Geometry check sheet. Reference: the model listing, model coordinates, mm. A direction names the side the tool comes from. Coordinates: 2 decimals unless noted, no trailing zeros. Write each loop counter-clockwise with the first axis right and the second up, starting at its lowest first coordinate (ties: lowest second). Pieces come first, ordered by that corner, then holes. Notation, with made-up numbers: (-1, -24) -> (14, -24) arc R36 cw to (14, 14) -> close; hole circle Ø2 at (-14.75, 61). An arc over 180 degrees is marked (long way). Use a Markdown table: item, result.
```python
from build123d import *

# Parameters (mm, degrees)
SKETCH_1_R              = 40
SKETCH_1_R_2            = 13.5
EXTRUDE_1_DEPTH         = 2
HOLE_WIZARD_M4_1_D      = 4.5
HOLE_WIZARD_5_4_5_4_1_D = 5.4
SKETCH_8_R              = 29.5
SKETCH_8_R_2            = 21.5
EXTRUDE_2_DEPTH         = 29
CUT_EXTRUDE_START       = -9
SKETCH_10_R             = 29.5
SKETCH_10_R_2           = 27.5
CUT_EXTRUDE_2_DEPTH     = 9
HOLE_WIZARD_M3_1_D      = 2.5
HOLE_WIZARD_M3_1_DEPTH  = 8.5
HOLE_WIZARD_M3_1_TIP    = 0.751075774


with BuildPart() as part:
    # 草图1 → 凸台-拉伸1 (new body)
    with BuildSketch(Plane.XY):
        Circle(SKETCH_1_R)
        Circle(SKETCH_1_R_2, mode=Mode.SUBTRACT)
    extrude(amount=EXTRUDE_1_DEPTH)

    # M4 间隙孔1 (through all)
    with Locations(Plane(origin=(-17.5, 0, 2), x_dir=(1, 0, 0), z_dir=(0, 0, 1))):
        with Locations((0, 0), (17.5, 17.5), (35, 0), (17.5, -17.5)):
            Hole(HOLE_WIZARD_M4_1_D / 2)

    # Ø5.4 (5.4) 直径孔1 (through all)
    with Locations(Plane(origin=(0, 0, 0), x_dir=(-1, 0, 0), z_dir=(0, 0, -1))):
        with Locations((-30.310889132, 17.5), (0, 35), (30.310889132, 17.5), (30.310889132, -17.5), (0, -35), (-30.310889132, -17.5)):
            Hole(HOLE_WIZARD_5_4_5_4_1_D / 2)

    # 草图8 → 凸台-拉伸2 (add)
    with BuildSketch(Plane(origin=(0, 0, 0), x_dir=(-1, 0, 0), z_dir=(0, 0, -1))):
        with Locations(Location((0, 0, 0), (0, 0, 180))):
            Circle(SKETCH_8_R)
        with Locations(Location((0, 0, 0), (0, 0, 180))):
            Circle(SKETCH_8_R_2, mode=Mode.SUBTRACT)
    extrude(amount=EXTRUDE_2_DEPTH)

    # 草图10 → 切除-拉伸2 (cut)
    with BuildSketch(Plane(origin=(0, 0, -29), x_dir=(-1, 0, 0), z_dir=(0, 0, -1)).offset(CUT_EXTRUDE_START)):
        with Locations(Location((0, 0, 0), (0, 0, 180))):
            Circle(SKETCH_10_R)
        Circle(SKETCH_10_R_2, mode=Mode.SUBTRACT)
    extrude(amount=CUT_EXTRUDE_2_DEPTH, mode=Mode.SUBTRACT)

    # M3 螺纹孔1
    with Locations(Plane(origin=(25, 0, -29), x_dir=(-1, 0, 0), z_dir=(0, 0, -1))):
        with Locations((0, 0), (25, 25), (50, 0), (25, -25)):
            Hole(HOLE_WIZARD_M3_1_D / 2, depth=HOLE_WIZARD_M3_1_DEPTH)
            with Locations((0, 0, -(HOLE_WIZARD_M3_1_DEPTH + HOLE_WIZARD_M3_1_TIP / 2))):  # 118° drill point
                Cone(0, HOLE_WIZARD_M3_1_D / 2, HOLE_WIZARD_M3_1_TIP, mode=Mode.SUBTRACT)


solid = part.part
```
Item 1: Depth check by flat-ended pin: P1, Ø5, axis at y = -21.5, z = -21, coming from the -X side; P2, Ø6, axis at x = 17.5, y = 0, coming from the -Z side; P3, Ø1.5, axis at y = -15, z = -10.5, coming from the -X side. Enter the tip coordinate at first touch or a pass-through.
Answer block:
| item | result |
|---|---|
| P1 | stops at x = -22.39 |
| P2 | stops at z = 0 |
| P3 | stops at x = -25.83 |
Item 2: Section check B-B on y = 34. Record the boundary of the cut face in (x, z).
Answer block:
| item | result |
|---|---|
| outline | (-21.07, 0) -> (-2.51, 0) -> (-2.51, 2) -> (-21.07, 2) -> close; (2.51, 0) -> (21.07, 0) -> (21.07, 2) -> (2.51, 2) -> close |
Item 3: Tool access check on faces 1 (the cylindrical face through (-23.845, -0.479, -24.69)), 2 (the flat face through (14.13, -16.42, -29)). Record the directions out of +Z, -Z, +X, -X, +Y, -Y that give a thin tool (end or side, any length) a straight path to the whole face; none if there is none.
Answer block:
| item | result |
|---|---|
| face 1 | -Z |
| face 2 | -Z, +X, -X, +Y, -Y |
Item 4: Thickness scan on L1, parallel to Y at x = 0, z = -26.5; L2, parallel to Y at x = 9.5, z = -13; L3, parallel to Y at x = 2, z = -21. Record the ranges inside material, lowest first. Write a range as [from, to].
Answer block:
| item | result |
|---|---|
| L1 | y = [-27.5, -26.25], [-23.75, -21.5], [21.5, 23.75], [26.25, 27.5] |
| L2 | y = [-27.93, -19.29], [19.29, 27.93] |
| L3 | y = [-27.43, -21.41], [21.41, 27.43] |
Item 5: Mould release check, pull along Y, two halves, no side actions. Record for faces 3 (the cylindrical face through (-28.9, -15.2, 1)), 4 (the flat face through (17, -8, 2)), 5 (the cylindrical face through (28.14, -8.86, -9.86)), 6 (the cylindrical face through (-2.93, -13.18, 0.99)): +Y half, -Y half, draft (parallel to the pull), parting line (faces both ways), or undercut.
Answer block:
| item | result |
|---|---|
| face 3 | undercut |
| face 4 | draft |
| face 5 | parting line |
| face 6 | undercut |
Item 6: Section check C-C on z = -11. Record the boundary of the cut face in (x, y), then the cut area to 3 significant figures.
Answer block:
| item | result |
|---|---|
| outline | circle Ø59 at (0, 0); hole circle Ø43 at (0, 0) |
| area | 1,280 mm^2 |
Item 7: Section check D-D on y = -17.5. Record the boundary of the cut face in (x, z), then the cut area to 3 significant figures.
Answer block:
| item | result |
|---|---|
| outline | (-35.97, 0) -> (-33.01, 0) -> (-33.01, 2) -> (-35.97, 2) -> close; (-27.61, 0) -> (-23.75, 0) -> (-23.75, -20) -> (-21.21, -20) -> (-21.21, -29) -> (-12.49, -29) -> (-12.49, 0) -> (-2.25, 0) -> (-2.25, 2) -> (-27.61, 2) -> close; (2.25, 0) -> (12.49, 0) -> (12.49, -29) -> (21.21, -29) -> (21.21, -20) -> (23.75, -20) -> (23.75, 0) -> (27.61, 0) -> (27.61, 2) -> (2.25, 2) -> close; (33.01, 0) -> (35.97, 0) -> (35.97, 2) -> (33.01, 2) -> close |
| area | 721 mm^2 |
Item 8: Section check A-A on x = -17.5. Record the boundary of the cut face in (y, z), then the cut area to 3 significant figures.
Answer block:
| item | result |
|---|---|
| outline | (-35.97, 0) -> (-23.75, 0) -> (-23.75, -20) -> (-21.21, -20) -> (-21.21, -29) -> (-12.49, -29) -> (-12.49, 0) -> (-2.25, 0) -> (-2.25, 2) -> (-35.97, 2) -> close; (2.25, 0) -> (12.49, 0) -> (12.49, -29) -> (21.21, -29) -> (21.21, -20) -> (23.75, -20) -> (23.75, 0) -> (35.97, 0) -> (35.97, 2) -> (2.25, 2) -> close |
| area | 742 mm^2 |
